from build123d import *

# Parameters (mm, degrees)
BOSS_EXTRUDE1_DEPTH = 3
BOSS_EXTRUDE2_START = 20
SKETCH2_R           = 8
BOSS_EXTRUDE2_DEPTH = 5
SKETCH3_R           = 5.5
CUT_EXTRUDE1_DEPTH  = 116.445427837


with BuildPart() as part:
    # Sketch1 → Boss-Extrude1 (new, symmetric)
    with BuildSketch(Plane(origin=(0, 0, 0), x_dir=(1, 0, 0), z_dir=(0, 1, 0))):
        with BuildLine():
            Line((-45, -57), (45, -57))
            ThreePointArc((45, -57), (48.535533906, -55.535533906), (50, -52))
            Line((50, -52), (50, 52))
            ThreePointArc((50, 52), (48.535533906, 55.535533906), (45, 57))
            Line((45, 57), (-45, 57))
            ThreePointArc((-45, 57), (-48.535533906, 55.535533906), (-50, 52))
            Line((-50, 52), (-50, -52))
            ThreePointArc((-50, -52), (-48.535533906, -55.535533906), (-45, -57))
        make_face()
    extrude(amount=BOSS_EXTRUDE1_DEPTH, both=True)

    # Sketch2 → Boss-Extrude2 (add)
    with BuildSketch(Plane.XY.offset(BOSS_EXTRUDE2_START)):
        with BuildLine():
            Line((-25, -3), (-25, -17.338880751))
            ThreePointArc((-25, -17.338880751), (-20.170076441, -54.275307328), (5.241257633, -81.512999419))
            ThreePointArc((5.241257633, -81.512999419), (25.119909898, -81.306146184), (35, -64.055423774))
            Line((35, -64.055423774), (35, -3))
            Line((35, -3), (-25, -3))
        make_face()
        with Locations((15, -64.055423774)):
            Circle(SKETCH2_R, mode=Mode.SUBTRACT)
    boss_extrude2 = extrude(amount=-BOSS_EXTRUDE2_DEPTH)

    # Mirror1: Boss-Extrude2 across plane
    add(boss_extrude2.mirror(Plane.XY))

    # Sketch3 → Cut-Extrude1 (cut, through all)
    with BuildSketch(Plane(origin=(0, 3, 0), x_dir=(1, 0, 0), z_dir=(0, 1, 0))):
        with Locations(Location((35.5, 42, 0), (0, 0, 270))):
            Circle(SKETCH3_R)
        with Locations(Location((-35.5, 42, 0), (0, 0, 270))):
            Circle(SKETCH3_R)
        with Locations(Location((-35.5, -42, 0), (0, 0, 270))):
            Circle(SKETCH3_R)
        with Locations(Location((35.5, -42, 0), (0, 0, 270))):
            Circle(SKETCH3_R)
    extrude(amount=-CUT_EXTRUDE1_DEPTH, mode=Mode.SUBTRACT)


solid = part.part
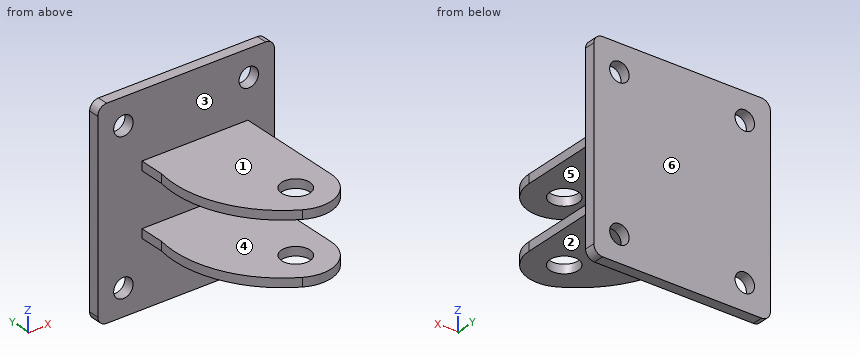
Can you work these out from the model? Positions are in its coordinate system, mm. Face numbers are marked on the shaded views. A direction names the side the tool comes from. Coordinates: 2 decimals unless noted, no trailing zeros. Loops run counter-clockwise (first coordinate to the right, second up) from the corner with the lowest first, then second, coordinate; pieces in that order, holes last. Notation, with made-up numbers: (64, 88) - (120, 88) arc R19 cw to (120, 112) - close; hole circle Ø11 at (83, -8). An arc over 180 degrees is marked (long way). Answer as a JSON object with one key per item and string values. Group by question number.
Item 1: On a 3-axis mill with a long thin cutter (end or side, diameter ignored), from which of +Z, -Z, +X, -X, +Y, -Y can I reach the whole of each face in a straight line? I mean the marked faces 5 and 6. Say none if no direction works.
Item 2: For pin 1 (1 mm diameter, centred on x = 2, y = -19, fed in from -Z); pin 2 (17.5 mm diameter, centred on x = -35.5, z = -42, fed in from -Y); pin 3 (5 mm diameter, centred on x = -15, y = -24.5, fed in from +Z); pin 4 (9 mm diameter, centred on x = 35.5, z = 42, fed in from -Y), each with a flat end and sliding along its axis, tell me the tip position at first contact or that it passes through.
Item 3: If we section it at B-B (x = -35.5): List the corners of the cut face in (y, z) for me.
Item 4: If we section it at D-D (z = -25.5): List the corners of the cut face in (x, y) for me, plus the area to 3 significant figures.
Item 5: If we mould it in two halves opening along Z, with no side actions, what happens to the marked faces 1, 2, 3 and 4? For each: released by +Z, released by -Z, zero draft, split by the parting line, or undercut.
Item 6: If I drill on L1, parallel to X at y = 1, z = 42; L2, parallel to Z at x = 18, y = -27.5; L3, parallel to Y at x = 15, z = 18.85, over which ranges is the centre line in solid material (lowest first)? Write a range as from..to.
Item 7: If we section it at A-A (y = -14.5): List the corners of the cut face in (x, z) for me.
Item 8: If we section it at C-C (z = -45.5): List the corners of the cut face in (x, y) for me.
Returned:
{
 "1": {"face 5": "+X, -X, -Y", "face 6": "+Z, -Z, +X, -X, +Y"},
 "2": {"pin 1": "stops at z = -20", "pin 2": "stops at y = -3", "pin 3": "stops at z = 20", "pin 4": "passes through"},
 "3": {"outline": "(-3, -57) - (3, -57) - (3, -47.5) - (-3, -47.5) - close; (-3, -36.5) - (3, -36.5) - (3, 36.5) - (-3, 36.5) - close; (-3, 47.5) - (3, 47.5) - (3, 57) - (-3, 57) - close"},
 "4": {"outline": "(-50, -3) - (50, -3) - (50, 3) - (-50, 3) - close", "area": "600 mm²"},
 "5": {"face 1": "released by +Z", "face 2": "released by -Z", "face 3": "undercut", "face 4": "undercut"},
 "6": {"L1": "x = -50..-41, -30..30, 41..50", "L2": "z = -20..-15, 15..20", "L3": "y = -84.06..-72.06, -56.06..3"},
 "7": {"outline": "(-25, -20) - (35, -20) - (35, -15) - (-25, -15) - close; (-25, 15) - (35, 15) - (35, 20) - (-25, 20) - close"},
 "8": {"outline": "(-50, -3) - (-39.74, -3) - (-39.74, 3) - (-50, 3) - close; (-31.26, -3) - (31.26, -3) - (31.26, 3) - (-31.26, 3) - close; (39.74, -3) - (50, -3) - (50, 3) - (39.74, 3) - close"}
}
